Could you check a few things on this model? Use its own coordinates, in mm. Face numbers are marked on the shaded views. A direction names the side the tool comes from. Coordinates: 2 decimals unless noted, no trailing zeros. Order: outer loops, then holes, each group sorted by start corner. A loop starts at its lowest first (then second) coordinate and runs counter-clockwise, first axis right, second up. Notation, with made-up numbers: (-14, 40.5) - (21, 40.5) arc R5 ccw to (21, 47.5) - close; hole circle Ø10 at (88.25, 0.25). An arc over 180 degrees is marked (long way). Answer as CSV lines item,"result". Start each with the question number.
1. I want a section at C-C, the plane x = 89. List the corners of the cut face in (y, z) for me, and give its area (3 significant figures).
2. I need wall thicknesses on probe 1 along X at (y, z) = (18, 36); probe 2 along Y at (x, z) = (83, 28); probe 3 along Z at (x, y) = (76, 15.5). Which ranges of each line are inside material? Lowest first, please.
3. I want a section at A-A, the plane z = 33.5. List the corners of the cut face in (x, y) for me, and give its area (3 significant figures).
4. For the marked faces 1, 2 and 3, which set-ups out of +Z, -Z, +X, -X, +Y, -Y let a thin tool reach every point of the face, with its end or its side?
5. For pin 1 (7 mm diameter, centred on y = 8.5, z = 34, fed in from +X); pin 2 (1.5 mm diameter, centred on x = 61, y = 36, fed in from +Z), each with a flat end and sliding along its axis, tell me the tip position at first contact or that it passes through.
6. I want a section at D-D, the plane y = 19. List the corners of the cut face in (x, z) for me.
7. I want a section at B-B, the plane y = 35.5. List the corners of the cut face in (x, z) for me, and give its area (3 significant figures).
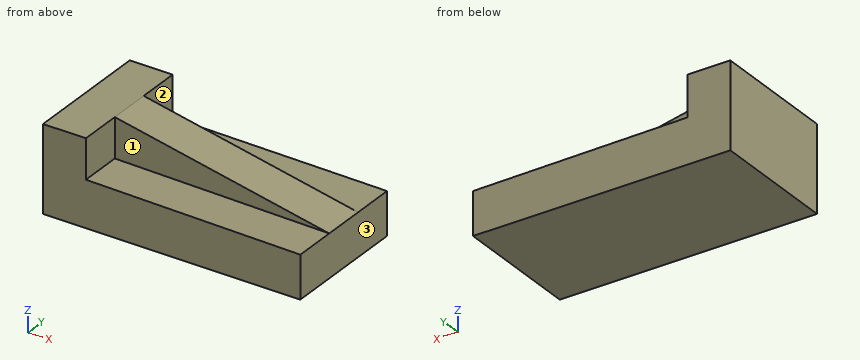
from build123d import *

# Parameters (mm, degrees)
F1_DEPTH = 76.2
F3_DEPTH = 76.2
F5_DEPTH = 25.4
F7_DEPTH = 25.4


with BuildPart() as f1:
    # F0 (on Front) → F1 (new body)
    with BuildSketch(Plane.XZ):
        Polygon((0, 50.8), (0, 0), (152.4, 0), (152.4, 25.4), (25.4, 25.4), (25.4, 50.8), align=None)
    extrude(amount=-F1_DEPTH)

    # F2 (on face) → F3 (join)
    with BuildSketch(Plane.XZ):
        Polygon((152.4, 25.4), (25.4, 50.8), (25.4, 25.4), align=None)
    extrude(amount=-F3_DEPTH)

    # F4 (on face) → F5 (cut)
    with BuildSketch(Plane.XZ):
        Polygon((152.4, 25.4), (25.4, 50.8), (25.4, 27.398381), align=None)
    extrude(amount=-F5_DEPTH, mode=Mode.SUBTRACT)

    # F6 (on face) → F7 (cut)
    with BuildSketch(Plane(origin=(0, 76.2, 0), x_dir=(-1, 0, 0), z_dir=(0, 1, 0))):
        Polygon((-25.4, 26.62628), (-25.4, 50.8), (-152.4, 25.4), align=None)
    extrude(amount=-F7_DEPTH, mode=Mode.SUBTRACT)


solid = f1.part
Solved:
1,outline,"(0, 0) - (76.2, 0) - (76.2, 26.01) - (50.8, 26.01) - (50.8, 38.08) - (25.4, 38.08) - (25.4, 26.4) - (0, 26.4) - close"
1,area,"2,300 mm2"
2,probe 1,"x = 0 to 25.4"
2,probe 2,"y = 25.4 to 50.8"
2,probe 3,"z = 0 to 26.6"
3,outline,"(0, 0) - (25.4, 0) - (25.4, 25.4) - (111.9, 25.4) - (111.9, 50.8) - (25.4, 50.8) - (25.4, 76.2) - (0, 76.2) - close"
3,area,"4,130 mm2"
4,face 1,"+Z, +X, -Y"
4,face 2,"+Z, +X, +Y"
4,face 3,"+Z, -Z, +X, +Y, -Y"
5,pin 1,"stops at x = 25.4"
5,pin 2,"stops at z = 43.83"
6,outline,"(0, 0) - (152.4, 0) - (152.4, 25.4) - (25.4, 27.4) - (25.4, 50.8) - (0, 50.8) - close"
7,outline,"(0, 0) - (152.4, 0) - (152.4, 25.4) - (25.4, 50.8) - (0, 50.8) - close"
7,area,"6,130 mm2"
